Design review of the part built by this model. Coordinates are the model's own, in mm. A direction names the side the tool comes from. Round coordinates to 2 decimals unless told otherwise and drop trailing zeros. Order: outer loops, then holes, each group sorted by start corner. A loop starts at its lowest first (then second) coordinate and runs counter-clockwise, first axis right, second up.
from build123d import *

# Parameters (mm, degrees)
BOSS_EXTRUDE1_REACH     = 167.297
SKETCH3_R               = 4
SKETCH4_R               = 1
CUT_EXTRUDE1_DEPTH      = 14
SKETCH5_R               = 1.5
CUT_EXTRUDE2_DEPTH      = 5.2
CUT_EXTRUDE3_DEPTH      = 129.074548772
CUT_EXTRUDE3_DEPTH_BACK = 129.074548772
SKETCH6_R               = 2.25


with BuildPart() as part:
    # Sketch2 → Revolve1 (revolve)
    with BuildSketch(Plane(origin=(0, 0, 0), x_dir=(0, 0, -1), z_dir=(1, 0, 0)), mode=Mode.PRIVATE) as revolve1_sk:
        with BuildLine():
            Line((95.3, 14.75), (95.3, 12.75))
            ThreePointArc((95.3, 12.75), (45.630862999, 19.624348561), (-0.05, 40.301354974))
            Line((-0.05, 40.301354974), (-0.05, 44.75))
            Line((-0.05, 44.75), (2.25, 44.75))
            Line((2.25, 44.75), (2.25, 49.75))
            Line((2.25, 49.75), (-0.35, 49.75))
            Line((-0.35, 49.75), (-0.35, 60))
            Line((-0.35, 60), (4.25, 60))
            Line((4.25, 60), (4.25, 40.301354974))
            ThreePointArc((4.25, 40.301354974), (48.016349969, 21.258883202), (95.3, 14.75))
        make_face()
    revolve(revolve1_sk.sketch.rotate(Axis((0, 0, 95.3), (0, 0, -1)), 180), axis=Axis((0, 0, 95.3), (0, 0, -1)))

    # Sketch3 → Boss-Extrude1 (add, up to next)
    with BuildSketch(Plane(origin=(0, 61, 0), x_dir=(-1, 0, 0), z_dir=(0, -1, 0)), mode=Mode.PRIVATE) as boss_extrude1_sk1:
        with Locations(Location((0, 4.25, 0), (0, 0, 180))):
            Circle(SKETCH3_R)
    boss_extrude1_tool1 = extrude(boss_extrude1_sk1.sketch, amount=BOSS_EXTRUDE1_REACH, mode=Mode.PRIVATE) - part.part
    add(boss_extrude1_tool1.solids().sort_by_distance((0, 61, -4.25))[0])

    # Sketch4 → Cut-Extrude1 (cut)
    with BuildSketch(Plane(origin=(0, 61, 0), x_dir=(1, 0, 0), z_dir=(0, 1, 0))):
        with Locations(Location((0, 4.25, 0), (0, 0, 180))):
            Circle(SKETCH4_R)
    extrude(amount=-CUT_EXTRUDE1_DEPTH, mode=Mode.SUBTRACT)

    # Sketch5 → Cut-Extrude2 (cut)
    with BuildSketch(Plane.XY):
        with Locations(Location((0, 46.797368966, 0), (0, 0, 77.98506808))):
            Circle(SKETCH5_R)
    extrude(amount=-CUT_EXTRUDE2_DEPTH, mode=Mode.SUBTRACT)

    # Sketch6 → Cut-Extrude3 (cut, two sides: drawn at the far end of the back side and taken through both)
    with BuildSketch(Plane.XY.offset(-CUT_EXTRUDE3_DEPTH_BACK)):
        with Locations((54, 0)):
            Circle(SKETCH6_R)
        with Locations((27, -46.765371804)):
            Circle(SKETCH6_R)
        with Locations((-27, -46.765371804)):
            Circle(SKETCH6_R)
        with Locations((-54, 0)):
            Circle(SKETCH6_R)
        with Locations((-27, 46.765371804)):
            Circle(SKETCH6_R)
        with Locations((27, 46.765371804)):
            Circle(SKETCH6_R)
    extrude(amount=CUT_EXTRUDE3_DEPTH + CUT_EXTRUDE3_DEPTH_BACK, mode=Mode.SUBTRACT)


solid = part.part
1) Take a section at C-C on z = -12.5. Give the boundary of the cut face in (x, y) (1 decimal).
Results:
outline: circle Ø71.2 at (0, 0); hole circle Ø66 at (0, 0)
2) Take a section at D-D on x = -27. State how many separate pieces and enclosed holes the cut face has, plus the area to 3 significant figures.
Results:
separate pieces: 3
enclosed holes: 0
area: 455 mm2
3) Take a section at A-A on y = 0. Give the boundary of the cut face in (x, z).
Results:
outline: (-60, -4.25) - (-56.25, -4.25) - (-56.25, 0.35) - (-60, 0.35) - close; (-51.75, -4.25) - (-40.3, -4.25) arc R175 cw to (-14.75, -95.3) - (-12.75, -95.3) arc R175 ccw to (-40.3, 0.05) - (-44.75, 0.05) - (-44.75, -2.25) - (-49.75, -2.25) - (-49.75, 0.35) - (-51.75, 0.35) - close; (12.75, -95.3) - (14.75, -95.3) arc R175 cw to (40.3, -4.25) - (51.75, -4.25) - (51.75, 0.35) - (49.75, 0.35) - (49.75, -2.25) - (44.75, -2.25) - (44.75, 0.05) - (40.3, 0.05) arc R175 ccw to start; (56.25, -4.25) - (60, -4.25) - (60, 0.35) - (56.25, 0.35) - close
4) The part is to be moulded in two halves that separate along X. For faces 4 (the face through (22, -45, 0.35)), 5 (the face through (28.04, 44.77, -1.98)), 6 (the face through (-0.867, 49.623, -8.155)), say which applies: released by +X, released by -X, zero draft, split by the parting line, or undercut.
Results:
face 4: zero draft
face 5: undercut
face 6: split by the parting line
5) Clearance check with flat-ended pins moving along their axes: P1, Ø0.9, axis at x = 0, y = 46.5, coming from the +Z side; P2, Ø6, axis at y = 13, z = -83.5, coming from the -X side; P3, Ø1.5, axis at x = 34.5, y = 27.5, coming from the -Z side. State where each tip first meets the part, or that it passes through.
Results:
P1: stops at z = -5.2
P2: stops at x = -11.39
P3: stops at z = -4.25
6) Take a section at B-B on x = -54. Give the boundary of the cut face in (y, z).
Results:
outline: (-26.15, -4.25) - (-2.25, -4.25) - (-2.25, 0.35) - (-26.15, 0.35) - close; (2.25, -4.25) - (26.15, -4.25) - (26.15, 0.35) - (2.25, 0.35) - close
7) For faces 1 (the face through (-56.248, 0.099, -1.982)), 2 (the face through (12, -39, -4.25)), 3 (the face through (-19, -41, -2.25)), list the 3-axis set-ups (+Z, -Z, +X, -X, +Y, -Y) from which the entire face can be reached by the end or side of a thin tool; tool diameter is ignored.
Results:
face 1: +Z, -Z
face 2: -Z
face 3: +Z
8) To check wall thickness, follow line 1 along Y through (x, z) = (-27, -1); line 2 along Y through (x, z) = (27, -2); line 3 along X through (y, z) = (0, -1.55). State the ranges of each line that lie inside material, in increasing order.
Results:
line 1: y = -53.58 to -49.02, -44.52 to -41.79, -35.69 to -29.02, 29.02 to 35.69, 41.79 to 44.52, 49.02 to 53.58
line 2: y = -53.58 to -49.02, -44.52 to -41.79, -35.69 to -28.16, 28.16 to 35.69, 41.79 to 44.52, 49.02 to 53.58
line 3: x = -60 to -56.25, -51.75 to -49.75, -44.75 to -39.29, 39.29 to 44.75, 49.75 to 51.75, 56.25 to 60
